```python
from build123d import *

# Parameters (mm, degrees)
BOSS_EXTRUDE1_DEPTH         = 3.75
BOLT_HOLE_REACH             = 26.729
SKETCH2_R                   = 1.6
BOLT_HOLE_DIRECTION_2_REACH = 26.729
BOSS_EXTRUDE2_START         = 5
BOSS_EXTRUDE2_DEPTH         = 5
CUT_EXTRUDE2_START          = 11
SKETCH4_R                   = 2.85
CUT_EXTRUDE2_DEPTH          = 3
SKETCH7_RX                  = 10
SKETCH7_RY                  = 5
SWEEP2_START                = 10.247926509
SWEEP2_DEPTH                = 2.568432868
SKETCH11_W                  = 7.251223943
SKETCH11_H                  = 3.177760732
CUT_EXTRUDE3_DEPTH          = 20
CUT_EXTRUDE5_START          = -2
CUT_EXTRUDE5_DEPTH          = 2.7
SKETCH13_R                  = 1.6
CUT_EXTRUDE6_DEPTH          = 2.7
CUT_EXTRUDE7_START          = -11
CUT_EXTRUDE7_DEPTH          = 10


# Read off the part's stored shape, not the designer's step: Sweep2
with BuildPart() as part:
    # Sketch1 → Boss-Extrude1 (new, symmetric)
    with BuildSketch(Plane.XY):
        with BuildLine():
            Line((-12.1, 0), (-14.051700625, -20))
            Line((-14.051700625, -20), (-10.051700625, -20))
            Line((-10.051700625, -20), (-8.425, -3.439385846))
            ThreePointArc((-8.425, -3.439385846), (0, 9.1), (8.425, -3.439385846))
            Line((8.425, -3.439385846), (10.051700625, -20))
            Line((10.051700625, -20), (14.051700625, -20))
            Line((14.051700625, -20), (12.1, 0))
            ThreePointArc((12.1, 0), (0, 12.1), (-12.1, 0))
        make_face()
    extrude(amount=BOSS_EXTRUDE1_DEPTH, both=True)

    # Bolt Hole: up to this plane
    bolt_hole_end = Plane(origin=(14.051700625, -20, 3.75), z_dir=(-0.995272319868323, -0.09712368044883128, 0))
    # Sketch2 → Bolt Hole (cut, up to the surface)
    with BuildSketch(Plane(origin=(0, 0, 0), x_dir=(0, 0, -1), z_dir=(1, 0, 0)), mode=Mode.PRIVATE) as bolt_hole_sk1:
        with Locations(Location((0, -10, 0), (0, 0, 90))):
            Circle(SKETCH2_R)
    bolt_hole_tool1 = split(extrude(bolt_hole_sk1.sketch, amount=BOLT_HOLE_REACH, mode=Mode.PRIVATE), bisect_by=bolt_hole_end, keep=Keep.BOTH, mode=Mode.PRIVATE)
    add(bolt_hole_tool1.solids().sort_by_distance((0, -10, 0))[0], mode=Mode.SUBTRACT)

    # Bolt Hole direction 2: up to this plane
    bolt_hole_direction_2_end = Plane(origin=(-12.1, 0, 3.75), z_dir=(0.995272319868323, -0.09712368044883138, 0))
    # Sketch2 → Bolt Hole direction 2 (cut, up to the surface)
    with BuildSketch(Plane(origin=(0, 0, 0), x_dir=(0, 0, -1), z_dir=(1, 0, 0)), mode=Mode.PRIVATE) as bolt_hole_direction_2_sk1:
        with Locations(Location((0, -10, 0), (0, 0, 90))):
            Circle(SKETCH2_R)
    bolt_hole_direction_2_tool1 = split(extrude(bolt_hole_direction_2_sk1.sketch, amount=-BOLT_HOLE_DIRECTION_2_REACH, mode=Mode.PRIVATE), bisect_by=bolt_hole_direction_2_end, keep=Keep.BOTH, mode=Mode.PRIVATE)
    add(bolt_hole_direction_2_tool1.solids().sort_by_distance((0, -10, 0))[0], mode=Mode.SUBTRACT)

    # Sketch3 → Boss-Extrude2 (add)
    with BuildSketch(Plane.XY.offset(3.75).offset(BOSS_EXTRUDE2_START)):
        with BuildLine():
            ThreePointArc((12.1, 0), (0, 12.1), (-12.1, 0))
            Line((-12.1, 0), (-6.05, 0))
            ThreePointArc((-6.05, 0), (0, 6.05), (6.05, 0))
            Line((6.05, 0), (12.1, 0))
        make_face()
        Polygon((-6.05, 0), (-12.1, 0), (-14.051700625, -20), (-8.001700625, -20), align=None)
        Polygon((14.051700625, -20), (12.1, 0), (6.05, 0), (8.001700625, -20), align=None)
    boss_extrude2 = extrude(amount=-BOSS_EXTRUDE2_DEPTH)

    # Sketch4 → Cut-Extrude2 (cut)
    with BuildSketch(Plane(origin=(0, 0, 0), x_dir=(0, 0, -1), z_dir=(1, 0, 0)).offset(CUT_EXTRUDE2_START)):
        with Locations(Location((0, -10, 0), (0, 0, 90))):
            Circle(SKETCH4_R)
    extrude(amount=CUT_EXTRUDE2_DEPTH, mode=Mode.SUBTRACT)

    # Sweep1: sweep along a path in Sketch8
    with BuildLine(Plane(origin=(0, 0, 0), x_dir=(0, 0, -1), z_dir=(1, 0, 0))) as sweep1_path:
        Line((20, 45), (0, 9.1))
    # Sketch7 → Sweep1 (sweep)
    with BuildSketch(Plane(origin=(0, 45, 0), x_dir=(1, 0, 0), z_dir=(0, 1, 0))):
        with Locations(Location((0, 20), (0, 0, -90))):
            Ellipse(SKETCH7_RX, SKETCH7_RY)
    sweep(path=sweep1_path.line)

    # Mirror2: Boss-Extrude2 across plane
    add(boss_extrude2.mirror(Plane.XY))

    # Sweep2 outline → Sweep2 (add)
    with BuildSketch(Plane(origin=(0, 0, 0), x_dir=(1, 0, 0), z_dir=(0, 0.8735827557825672, -0.48667562996243774)).offset(SWEEP2_START)):
        with BuildLine():
            add(Edge.make_bspline(
                [(-2.420614591, 3.21510088), (-4.140808386, 1.552228138), (-6.669000046, -3.159441487), (-5.965430129, -9.385769202), (-3.27241307, -12.380396445), (-1.32464484, -13.16457579), (1.32464484, -13.16457579), (3.27241307, -12.380396445), (5.965430129, -9.385769202), (6.669000046, -3.159441487), (4.140808386, 1.552228138), (1.714602002, 3.897587408), (0.891272318, 4.380182485), (0, 4.554319728), (-0.891272318, 4.380182485), (-1.714602002, 3.897587408), (-2.420614591, 3.21510088)],
                knots=[0.602606548, 0.602606548, 0.602606548, 0.602606548, 0.602606548, 0.602606548, 0.602606548, 1, 1, 1, 1, 1, 1.397393452, 1.397393452, 1.397393452, 1.397393452, 1.397393452, 1.560494133, 1.560494133, 1.560494133, 1.560494133, 1.560494133, 1.560494133, 1.560494133], degree=6, weights=[1, 1, 0.816743691, 0.81626183, 0.938272083, 1, 1, 0.938272083, 0.81626183, 0.816743691, 1, 1, 0.995833333, 0.99375, 0.995833333, 1, 1]))
        make_face()
    extrude(amount=SWEEP2_DEPTH)

    # Sketch11 → Cut-Extrude3 (cut)
    with BuildSketch(Plane(origin=(0, 0, 0), x_dir=(1, 0, 0), z_dir=(0, 1, 0))):
        with Locations((-0.008642554, -10.338880366)):
            Rectangle(SKETCH11_W, SKETCH11_H)
    extrude(amount=CUT_EXTRUDE3_DEPTH, mode=Mode.SUBTRACT)

    # Sketch12 → Cut-Extrude5 (cut)
    with BuildSketch(Plane(origin=(0, 45, 0), x_dir=(1, 0, 0), z_dir=(0, 1, 0)).offset(CUT_EXTRUDE5_START)):
        Polygon((-3.290892766, 20.010039827), (-3.290892766, 22.85), (3.290892766, 22.85), (3.290892766, 20.010039827), (1.642548134, 17.155023177), (-1.642548134, 17.155023177), align=None)
    extrude(amount=-CUT_EXTRUDE5_DEPTH, mode=Mode.SUBTRACT)

    # Sketch13 → Cut-Extrude6 (cut)
    with BuildSketch(Plane(origin=(0, 45, 0), x_dir=(1, 0, 0), z_dir=(0, 1, 0))):
        with Locations(Location((0, 20, 0), (0, 0, 270))):
            Circle(SKETCH13_R)
    extrude(amount=-CUT_EXTRUDE6_DEPTH, mode=Mode.SUBTRACT)

    # Sketch14 → Cut-Extrude7 (cut)
    with BuildSketch(Plane(origin=(0, 0, 0), x_dir=(0, 0, -1), z_dir=(1, 0, 0)).offset(CUT_EXTRUDE7_START)):
        Polygon((-3.233161507, -10), (-1.616580754, -12.8), (1.616580754, -12.8), (3.233161507, -10), (1.616580754, -7.2), (-1.616580754, -7.2), align=None)
    extrude(amount=-CUT_EXTRUDE7_DEPTH, mode=Mode.SUBTRACT)


solid = part.part
```
CAD build for the part. Positions are in the model's coordinates, mm. A direction names the side the tool comes from. Coordinates: 2 decimals unless noted, no trailing zeros. Write each loop counter-clockwise with the first axis right and the second up, starting at its lowest first coordinate (ties: lowest second). Pieces come first, ordered by that corner, then holes. Notation, with made-up numbers: (-31, 27.5) -> (-4, 27.5) arc R24 cw to (-4, 45.5) -> close; hole circle Ø9 at (38, 39). An arc over 180 degrees is marked (long way). Use CSV: the item, a comma, the result in double quotes. Start each with the question number.
Item 1: Band-saw the part on D-D, the plane y = -13.5. Write the cut outline in (x, z).
Item 2: Band-saw the part on B-B, the plane x = 7.25. Write the cut outline in (y, z).
Item 3: Band-saw the part on C-C, the plane z = 0. Give the number of separate pieces and of enclosed holes in the cut face, plus the area to 3 significant figures.
Item 4: Band-saw the part on A-A, the plane y = 5. Write the cut outline in (x, z), plus the area to 3 significant figures.
Item 5: Two-plate mould, pull along X, no slides. Class faces 4 (the flat face through (-6.4, -0.2, 8.75)), 5 (the cylindrical face through (7.98, 9.096, -0.123)), 6 (the flat face through (-9.25, -11.84, 0.05)): +X half, -X half, draft (parallel to the pull), parting line (faces both ways), or undercut.
Item 6: Drop flat-ended pins along their axis: P1, Ø4, axis at x = -8.5, y = -8.5, coming from the -Z side; P2, Ø1.4, axis at y = 41.5, z = -21.5, coming from the +X side; P3, Ø2, axis at x = 0, y = 41.5, coming from the -Z side. Give the stop position or say it passes through.
Item 7: Wall check: probe 1 along Z at (x, y) = (10, -10); probe 2 along X at (y, z) = (-15.5, -4); probe 3 along X at (y, z) = (-2, -8.5). Give the ranges that are in metal, low to high.
Item 8: Tool access for faces 1 (the flat face through (2.478, 41.669, -18.603)), 2 (the flat face through (-12, -7.2, 0)), 3 (the flat face through (9.227, -11.604, 0.886)): list every direction of +Z, -Z, +X, -X, +Y, -Y with a clear straight run to the whole face (end or side of a thin tool).
Response values:
1,outline,"(-13.42, -8.75) -> (-7.37, -8.75) -> (-7.37, -3.75) -> (-9.41, -3.75) -> (-9.41, 3.75) -> (-7.37, 3.75) -> (-7.37, 8.75) -> (-13.42, 8.75) -> close; (7.37, -8.75) -> (13.42, -8.75) -> (13.42, 8.75) -> (7.37, 8.75) -> (7.37, 3.75) -> (9.41, 3.75) -> (9.41, -3.75) -> (7.37, -3.75) -> close"
2,outline,"(-12.3, -8.75) -> (9.69, -8.75) -> (9.69, 8.75) -> (-12.3, 8.75) -> (-12.3, 3.75) -> (5.5, 3.75) -> (5.5, -3.75) -> (-12.3, -3.75) -> close"
3,separate pieces,"3"
3,enclosed holes,"0"
3,area,"335 mm2"
4,outline,"(-11.02, -8.75) -> (-3.41, -8.75) -> (-3.41, -3.75) -> (-7.6, -3.75) -> (-7.6, 3.75) -> (-3.41, 3.75) -> (-3.41, 8.75) -> (-11.02, 8.75) -> close; (3.41, -8.75) -> (11.02, -8.75) -> (11.02, 8.75) -> (3.41, 8.75) -> (3.41, 3.75) -> (7.6, 3.75) -> (7.6, -3.75) -> (3.41, -3.75) -> close"
4,area,"203 mm2"
5,face 4,"draft"
5,face 5,"parting line"
5,face 6,"undercut"
6,P1,"stops at z = -8.75"
6,P2,"stops at x = 4.82"
6,P3,"stops at z = -28.61"
7,probe 1,"z = -8.75 to -1.6, 1.6 to 8.75"
7,probe 2,"x = -13.61 to -7.56, 7.56 to 13.61"
7,probe 3,"x = -12.3 to -6.25, 6.25 to 12.3"
8,face 1,"none"
8,face 2,"-X"
8,face 3,"-Y"
